Can you work these out from the drawing? Everything is in mm from the part's minimum corner. A direction names the side the tool comes from. Round coordinates to 2 decimals unless told otherwise and drop trailing zeros. Write each loop counter-clockwise with the first axis right and the second up, starting at its lowest first coordinate (ties: lowest second). Pieces come first, ordered by that corner, then holes.
Q1. Please list where these lines run through material, in increasing order: line 1 along Y through (x, z) = (23, 19.5); line 2 along Z through (x, y) = (7.75, 17.8); line 3 along X through (y, z) = (14, 4.5).
Q2. If we section it at A-A (x = 25.5): Please give me the cut outline in (y, z), plus the area to 3 significant figures.
Q3. If we section it at B-B (x = 9.5): Please give me the cut outline in (y, z).
Q4. We'd pull the mould along Y, two halves only. Please class the marked faces 4, 5, 6 and 7: +Y half, -Y half, draft (parallel to the pull), parting line (faces both ways), or undercut.
Q5. I'm going to push flat-ended pins straight in: pin 1 Ø8 at (y, z) = (16, 14) entering from +X; pin 2 Ø7.5 at (x, y) = (35, 31.5) entering from -Z; pin 3 Ø1 at (x, z) = (45, 14.5) entering from +Y. Where does each tip first touch, or does it pass through?
Q6. If we section it at D-D (y = 27.5): Please give me the cut outline in (x, z), plus the area to 3 significant figures.
Q7. For the marked faces 1, 2 and 3, which set-ups out of +Z, -Z, +X, -X, +Y, -Y let a thin tool reach every point of the face, with its end or its side?
Q8. If we section it at C-C (z = 2.5): Please give me the cut outline in (x, y), plus the area to 3 significant figures.
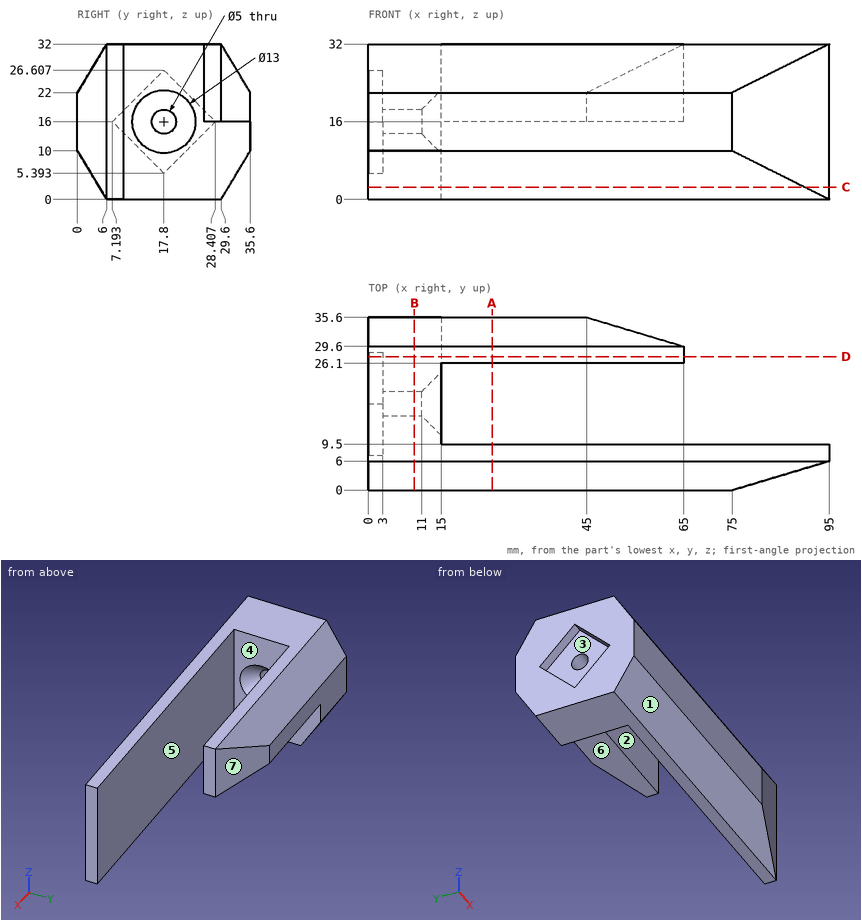
A:
1. line 1: y = 0 to 9.5, 26.1 to 35.6
1. line 2: z = 0 to 13.5, 18.5 to 32
1. line 3: x = 0 to 15
2. outline: (0, 10) - (6, 0) - (9.5, 0) - (9.5, 32) - (6, 32) - (0, 22) - close; (26.1, 16) - (35.6, 16) - (35.6, 22) - (29.6, 32) - (26.1, 32) - close
2. area: 366 mm2
3. outline: (0, 10) - (6, 0) - (29.6, 0) - (35.6, 10) - (35.6, 22) - (29.6, 32) - (6, 32) - (0, 22) - close; hole circle Ø5 at (17.8, 16)
4. face 4: undercut
4. face 5: undercut
4. face 6: draft
4. face 7: +Y half
5. pin 1: stops at x = 15
5. pin 2: stops at z = 16
5. pin 3: stops at y = 9.5
6. outline: (0, 0) - (15, 0) - (15, 16) - (65, 16) - (65, 32) - (0, 32) - (0, 16.91) - (3, 16.91) - (3, 15.09) - (0, 15.09) - close
6. area: 1,270 mm2
7. face 1: -Z, +X, -X, -Y
7. face 2: +Z, -Z, +X
7. face 3: -X
8. outline: (0, 4.5) - (90, 4.5) - (95, 6) - (95, 9.5) - (15, 9.5) - (15, 31.1) - (0, 31.1) - close
8. area: 795 mm2
